CAD build for the part. Positions are in the model's coordinates, mm. Face numbers are marked on the shaded views. Coordinates: 2 decimals unless noted, no trailing zeros. Write each loop counter-clockwise with the first axis right and the second up, starting at its lowest first coordinate (ties: lowest second). Pieces come first, ordered by that corner, then holes. Notation, with made-up numbers: M 28.25,1 L 63.25,1 A14 ccw 63.25,19 Z; hole C -17.5,85.25 d7. An arc over 180 degrees is marked long. Put each result on its own line as item: value. Start each with the question number.
```python
from build123d import *

# Parameters (mm, degrees)
ESQUISSE1_W             = 20
ESQUISSE1_H             = 70
ESQUISSE1_R             = 1.75
BOSS_EXTRU_1_DEPTH      = 3
ESQUISSE2_R             = 1.75
BOSS_EXTRU_2_DEPTH      = 5
ESQUISSE3_R             = 1.1
ENL_V_MAT_EXTRU_1_DEPTH = 5
CONG_1_R                = 5
CONG_2_R                = 0.5


with BuildPart() as part:
    # Esquisse1 → Boss.-Extru.1 (new body)
    # profile 1 of 9: a face of its own
    with BuildSketch(Plane.XY):
        with Locations((10, 35)):
            Rectangle(ESQUISSE1_W, ESQUISSE1_H)
        with Locations((17, 3.5)):
            Circle(ESQUISSE1_R, mode=Mode.SUBTRACT)
        with Locations((3, 3.5)):
            Circle(ESQUISSE1_R, mode=Mode.SUBTRACT)
        with Locations((17, 19.5)):
            Circle(ESQUISSE1_R, mode=Mode.SUBTRACT)
        with Locations((3, 19.5)):
            Circle(ESQUISSE1_R, mode=Mode.SUBTRACT)
        with Locations((17, 50.5)):
            Circle(ESQUISSE1_R, mode=Mode.SUBTRACT)
        with Locations((3, 50.5)):
            Circle(ESQUISSE1_R, mode=Mode.SUBTRACT)
        with Locations((17, 66.5)):
            Circle(ESQUISSE1_R, mode=Mode.SUBTRACT)
        with Locations((3, 66.5)):
            Circle(ESQUISSE1_R, mode=Mode.SUBTRACT)
    # profile 2 of 9: a face of its own
    with BuildSketch(Plane.XY):
        with Locations((3, 66.5)):
            Circle(ESQUISSE1_R)
    # profile 3 of 9: a face of its own
    with BuildSketch(Plane.XY):
        with Locations((17, 66.5)):
            Circle(ESQUISSE1_R)
    # profile 4 of 9: a face of its own
    with BuildSketch(Plane.XY):
        with Locations((17, 50.5)):
            Circle(ESQUISSE1_R)
    # profile 5 of 9: a face of its own
    with BuildSketch(Plane.XY):
        with Locations((3, 50.5)):
            Circle(ESQUISSE1_R)
    # profile 6 of 9: a face of its own
    with BuildSketch(Plane.XY):
        with Locations((3, 19.5)):
            Circle(ESQUISSE1_R)
    # profile 7 of 9: a face of its own
    with BuildSketch(Plane.XY):
        with Locations((17, 19.5)):
            Circle(ESQUISSE1_R)
    # profile 8 of 9: a face of its own
    with BuildSketch(Plane.XY):
        with Locations((17, 3.5)):
            Circle(ESQUISSE1_R)
    # profile 9 of 9: a face of its own
    with BuildSketch(Plane.XY):
        with Locations((3, 3.5)):
            Circle(ESQUISSE1_R)
    extrude(amount=BOSS_EXTRU_1_DEPTH)

    # Esquisse2 → Boss.-Extru.2 (add)
    with BuildSketch(Plane(origin=(0, 0, 0), x_dir=(-1, 0, 0), z_dir=(0, 0, -1))):
        with Locations(Location((-17, 66.5, 0), (0, 0, 180))):
            Circle(ESQUISSE2_R)
        with Locations(Location((-3, 66.5, 0), (0, 0, 180))):
            Circle(ESQUISSE2_R)
        with Locations(Location((-17, 50.5, 0), (0, 0, 180))):
            Circle(ESQUISSE2_R)
        with Locations(Location((-3, 50.5, 0), (0, 0, 180))):
            Circle(ESQUISSE2_R)
        with Locations(Location((-17, 19.5, 0), (0, 0, 180))):
            Circle(ESQUISSE2_R)
        with Locations(Location((-3, 19.5, 0), (0, 0, 180))):
            Circle(ESQUISSE2_R)
        with Locations(Location((-17, 3.5, 0), (0, 0, 180))):
            Circle(ESQUISSE2_R)
        with Locations(Location((-3, 3.5, 0), (0, 0, 180))):
            Circle(ESQUISSE2_R)
    extrude(amount=BOSS_EXTRU_2_DEPTH)

    # Esquisse3 → Enl_v. mat.-Extru.1 (cut)
    with BuildSketch(Plane.XY.offset(3)):
        with Locations((2, 11.557756062)):
            Circle(ESQUISSE3_R)
        with Locations((2, 15.557756062)):
            Circle(ESQUISSE3_R)
        with Locations((2, 27.557756062)):
            Circle(ESQUISSE3_R)
        with Locations((2, 31.557756062)):
            Circle(ESQUISSE3_R)
        with Locations((2, 35.557756062)):
            Circle(ESQUISSE3_R)
        with Locations((18, 43.557756062)):
            Circle(ESQUISSE3_R)
        with Locations((18, 39.557756062)):
            Circle(ESQUISSE3_R)
        with Locations((18, 31.557756062)):
            Circle(ESQUISSE3_R)
        with Locations((18, 27.557756062)):
            Circle(ESQUISSE3_R)
        with Locations((18, 23.557756062)):
            Circle(ESQUISSE3_R)
        with Locations((18, 15.557756062)):
            Circle(ESQUISSE3_R)
        with Locations((18, 11.557756062)):
            Circle(ESQUISSE3_R)
        with BuildLine():
            ThreePointArc((11.1, 3.557756062), (10.777817459, 4.335573521), (10, 4.657756062))
            Line((10, 4.657756062), (10, 2.457756062))
            ThreePointArc((10, 2.457756062), (10.777817459, 2.779938602), (11.1, 3.557756062))
        make_face()
        with BuildLine():
            Line((10, 2.457756062), (10, 4.657756062))
            ThreePointArc((10, 4.657756062), (8.9, 3.557756062), (10, 2.457756062))
        make_face()
        with Locations((2, 23.557756062)):
            Circle(ESQUISSE3_R)
        with Locations((2, 47.557756062)):
            Circle(ESQUISSE3_R)
        with Locations((2, 43.557756062)):
            Circle(ESQUISSE3_R)
        with Locations((2, 39.557756062)):
            Circle(ESQUISSE3_R)
        with Locations((2, 55.557756062)):
            Circle(ESQUISSE3_R)
        with Locations((2, 59.557756062)):
            Circle(ESQUISSE3_R)
        with Locations((18, 59.557756062)):
            Circle(ESQUISSE3_R)
        with Locations((18, 47.557756062)):
            Circle(ESQUISSE3_R)
        with Locations((18, 35.557756062)):
            Circle(ESQUISSE3_R)
        with Locations((10, 7.557756062)):
            Circle(ESQUISSE3_R)
        with Locations((10, 11.557756062)):
            Circle(ESQUISSE3_R)
        with Locations((10, 15.557756062)):
            Circle(ESQUISSE3_R)
        with Locations((10, 19.557756062)):
            Circle(ESQUISSE3_R)
        with Locations((10, 23.557756062)):
            Circle(ESQUISSE3_R)
        with Locations((10, 27.557756062)):
            Circle(ESQUISSE3_R)
        with Locations((10, 31.557756062)):
            Circle(ESQUISSE3_R)
        with Locations((10, 35.557756062)):
            Circle(ESQUISSE3_R)
        with Locations((10, 39.557756062)):
            Circle(ESQUISSE3_R)
        with Locations((10, 43.557756062)):
            Circle(ESQUISSE3_R)
        with Locations((10, 47.557756062)):
            Circle(ESQUISSE3_R)
        with Locations((10, 51.557756062)):
            Circle(ESQUISSE3_R)
        with Locations((10, 55.557756062)):
            Circle(ESQUISSE3_R)
        with Locations((10, 59.557756062)):
            Circle(ESQUISSE3_R)
        with Locations((10, 63.557756062)):
            Circle(ESQUISSE3_R)
        with Locations((10, 67.557756062)):
            Circle(ESQUISSE3_R)
        with Locations((18, 55.557756062)):
            Circle(ESQUISSE3_R)
    extrude(amount=-ENL_V_MAT_EXTRU_1_DEPTH, mode=Mode.SUBTRACT)

    # Cong_1
    cong_1_edges = [part.edges().sort_by_distance(p)[0] for p in [
        (0, 0, 1.5),
        (0, 70, 1.5),
        (20, 70, 1.5),
        (20, 0, 1.5),
    ]]
    fillet(cong_1_edges, radius=CONG_1_R)

    # Cong_2
    cong_2_edges = [part.edges().sort_by_distance(p)[0] for p in [
        (10, 70, 0),
        (10, 70, 3),
        (10, 0, 0),
        (0, 35, 0),
        (20, 35, 0),
        (1.464466094, 68.535533906, 0),
        (1.464466094, 1.464466094, 0),
        (18.535533906, 1.464466094, 0),
        (18.535533906, 68.535533906, 0),
        (20, 35, 3),
        (10, 0, 3),
        (0, 35, 3),
        (1.464466094, 68.535533906, 3),
        (1.464466094, 1.464466094, 3),
        (18.535533906, 1.464466094, 3),
        (18.535533906, 68.535533906, 3),
    ]]
    fillet(cong_2_edges, radius=CONG_2_R)


solid = part.part
```
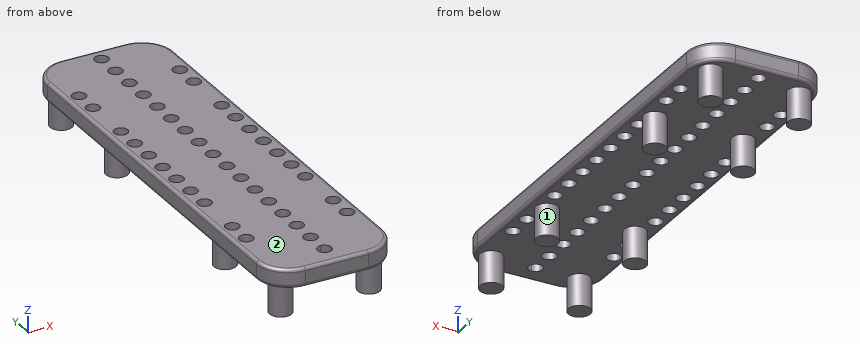
(1) Slice it at C-C, the plane x = 2. State how many separate pieces and enclosed holes the cut face has, then the cut area to 3 significant figures.
(2) Drop a flat-ended pin along its axis: pin 1 (3 mm diameter, centred on x = 8.5, y = 38.5, fed in from -Z). Give the stop position or say it passes through.
(3) Drill centre lines: line 1 (X direction, y = 36.5, z = 1.5); line 2 (Z direction, x = 6.5, y = 57.5); line 3 (Y direction, x = 16.75, z = -4). Where is each one in solid material? Low to high. Write a range as [from, to].
(4) Two-plate mould, pull along X, no slides. Class the marked faces 1 and 2: +X half, -X half, draft (parallel to the pull), parting line (faces both ways), or undercut.
(5) Slice it at B-B, the plane x = 13.5. Write the cut outline in (y, z).
(6) Slice it at A-A, the plane z = -3. Write the cut outline in (x, y).
Result set:
1. separate pieces: 12
1. enclosed holes: 0
1. area: 189 mm^2
2. pin 1: stops at z = 0
3. line 1: x = [0, 1.43], [2.57, 9.43], [10.57, 17.43], [18.57, 20]
3. line 2: z = [0, 3]
3. line 3: y = [1.77, 5.23], [17.77, 21.23], [48.77, 52.23], [64.77, 68.23]
4. face 1: undercut
4. face 2: draft
5. outline: M 0,0.5 A0.5 ccw 0.5,0 L 69.5,0 A0.5 ccw 70,0.5 L 70,2.5 A0.5 ccw 69.5,3 L 0.5,3 A0.5 ccw 0,2.5 Z
6. outline: C 3,3.5 d3.5; C 3,19.5 d3.5; C 3,50.5 d3.5; C 3,66.5 d3.5; C 17,3.5 d3.5; C 17,19.5 d3.5; C 17,50.5 d3.5; C 17,66.5 d3.5
